from build123d import *

# Parameters (mm, degrees)
F1_DEPTH = 6.35
F2_R     = 1.35255
F3_DEPTH = 4.7625
F4_R     = 1.35255
F5_DEPTH = 4.7625
F6_W     = 53.975
F6_H     = 1.5875
F7_DEPTH = 99.4996370206
F8_SIZE  = 1.58749


# Not quite as in the source:
# - a fillet or chamfer is up to 0.001 mm smaller than in the source, because OpenCascade refuses the exact size


with BuildPart() as f1:
    # F0 (on Top) → F1 (new body)
    with BuildSketch(Plane.XY):
        Polygon((0, -66.675), (0, 0), (-6.35, 0), (-99.4986370206, -60.325), (-99.4986370206, -66.675), align=None)
    extrude(amount=F1_DEPTH)

    # F2 (on face) → F3 (cut)
    with BuildSketch(Plane.YZ):
        with Locations((-63.5, 3.175)):
            Circle(F2_R)
        with Locations((-3.175, 3.175)):
            Circle(F2_R)
    extrude(amount=-F3_DEPTH, mode=Mode.SUBTRACT)

    # F4 (on face) → F5 (cut)
    with BuildSketch(Plane.XZ.offset(66.675)):
        with Locations((-96.3236370206, 3.175)):
            Circle(F4_R)
        with Locations((-9.525, 3.175)):
            Circle(F4_R)
    extrude(amount=-F5_DEPTH, mode=Mode.SUBTRACT)

    # F6 (on face) → F7 (cut, through all)
    with BuildSketch(Plane.YZ):
        with Locations((-33.3375, 5.55625)):
            Rectangle(F6_W, F6_H)
        with Locations((-33.3375, 0.79375)):
            Rectangle(F6_W, F6_H)
    extrude(amount=-F7_DEPTH, mode=Mode.SUBTRACT)

    # F8 (size 1.5875 in the source; OpenCascade refuses exactly that, so slightly less here)
    f8_edges = [f1.edges().sort_by_distance(p)[0] for p in [
        (-49.749319, -60.325, 4.7625),
        (-49.749319, -60.325, 1.5875),
        (-8.07756, -6.35, 4.7625),
        (-8.07756, -6.35, 1.5875),
    ]]
    chamfer(f8_edges, length=F8_SIZE)


solid = f1.part
Verification items for the finished model (mm, model axes). A direction names the side the tool comes from. Give positions to 0.01 mm unless a question says otherwise; leave off trailing zeros. Loops run counter-clockwise (first coordinate to the right, second up) from the corner with the lowest first, then second, coordinate; pieces in that order, holes last.
1) Thickness scan on line 1 along Z through (x, y) = (-8, -55); line 2 along Y through (x, z) = (-15, 1) (3 decimals); line 3 along X through (y, z) = (-63, 3.75). Record the ranges inside material, lowest first.
2) Sectioned sample at C-C, the plane y = -13.5. Enter the section's corners in (x, z).
3) Sectioned sample at A-A, the plane y = -63.5. Count the separate pieces of the cut face and the enclosed holes in it, then the cut area to 3 significant figures.
4) Depth check by flat-ended pin: pin 1 Ø6 at (x, y) = (-51.5, -35.5) entering from +Z; pin 2 Ø12 at (x, y) = (-37.5, -59) entering from -Z; pin 3 Ø0.8 at (x, z) = (-10, 3.5) entering from -Y; pin 4 Ø2 at (x, y) = (-38, -58) entering from +Z (3 decimals). Enter the tip coordinate at first touch or a pass-through.
5) Set-up check for faces 4 (the cylindrical face through (-2.35, -62.21, 3.58)), 5 (the flat face through (-37, -39, 1.588)), 6 (the flat face through (-96, -61.912, 3)): record each of +Z, -Z, +X, -X, +Y, -Y from which the full face is reachable in a straight line by a thin tool's end or side.
6) Draft check along Z on faces 1 (the flat face through (-37, -39, 4.762)), 2 (the cylindrical face through (-8.235, -64.327, 3.581)), 3 (the flat face through (0, -34, 3)). Enter one of: pulls with the +Z half, pulls with the -Z half, needs draft (parallel to the pull), parting line crosses it, or undercut.
Answers:
1. line 1: z = 1.59 to 4.76
1. line 2: y = -66.675 to -59.325, -7.35 to -5.602
1. line 3: x = -99.5 to -97.55, -95.1 to -10.75, -8.3 to -4.76
2. outline: (-27.2, 1.59) - (0, 1.59) - (0, 4.76) - (-27.2, 4.76) - close
3. separate pieces: 1
3. enclosed holes: 2
3. area: 607 mm2
4. pin 1: stops at z = 4.76
4. pin 2: stops at z = 0
4. pin 3: stops at y = -61.91
4. pin 4: stops at z = 5.025
5. face 4: +X
5. face 5: -Z, +X, -X
5. face 6: -Y
6. face 1: pulls with the +Z half
6. face 2: undercut
6. face 3: needs draft
